from build123d import *

# Parameters (mm, degrees)
F0_R     = 10.0711
F0_R_2   = 9.0551
F1_DEPTH = 1.27
F2_R     = 0.50799


# Not quite as in the source:
# - a fillet or chamfer is up to 0.001 mm smaller than in the source, because OpenCascade refuses the exact size


with BuildPart() as f1:
    # F0 (on Front) → F1 (new body, symmetric)
    with BuildSketch(Plane.XZ):
        Circle(F0_R)
        Circle(F0_R_2, mode=Mode.SUBTRACT)
    extrude(amount=F1_DEPTH, both=True)

    # F2 (radius 0.508 in the source; OpenCascade refuses exactly that, so slightly less here)
    f2_edges = [f1.edges().sort_by_distance(p)[0] for p in [
        (-9.0551, -1.27, 0),
        (-9.0551, 1.27, 0),
        (-10.0711, -1.27, 0),
        (-10.0711, 1.27, 0),
        (10.0711, 0, 0),
    ]]
    fillet(f2_edges, radius=F2_R)


solid = f1.part
The model under review builds one solid part; all positions refer to its coordinate system, in mm. Round coordinates to 2 decimals unless told otherwise and drop trailing zeros. Order: outer loops, then holes, each group sorted by start corner. A loop starts at its lowest first (then second) coordinate and runs counter-clockwise, first axis right, second up. Notation, with made-up numbers: (-32.75, 69.25) - (-15.75, 69.25) arc R38 cw to (-15.75, 108.25) - close; hole circle Ø6 at (-39.75, -37.75). An arc over 180 degrees is marked (long way). Use one line per item in the form item = value.
Q1. Mouldability with a two-part tool opening along Z and no side actions: class faces 1 (the cylindrical face through (-1.96, 0.01, -8.84)), 2 (the cylindrical face through (-1.311, -0.011, 9.985)) as pulls with the +Z half, pulls with the -Z half, needs draft (parallel to the pull), parting line crosses it, or undercut.
Response values:
face_1 = undercut
face_2 = parting line crosses it
Q2. Add section C-C on y = -0.05. Give the boundary of the cut face in (x, z), then the cut area to 3 significant figures.
Response values:
outline = circle Ø20.14 at (0, 0); hole circle Ø18.11 at (0, 0)
area = 61.0 mm^2
Q3. To check wall thickness, follow line 1 (Z direction, x = 0, y = 0.1); line 2 (X direction, y = -0.4, z = -6.25); line 3 (Z direction, x = 7, y = 0.7). State the ranges of each line that lie inside material, in increasing order.
Response values:
line_1 = -10.07 to -9.06, 9.06 to 10.07
line_2 = -7.9 to -6.55, 6.55 to 7.9
line_3 = -7.24 to -5.74, 5.74 to 7.24
Q4. Clearance check with flat-ended pins moving along their axes: P1, Ø1.5, axis at y = 0.5, z = 7.5, coming from the -X side; P2, Ø1.5, axis at x = -7, y = 0.5, coming from the +Z side; P3, Ø3, axis at x = 4, z = -5, coming from the +Y side; P4, Ø1, axis at y = -1, z = 7, coming from the +X side. State where each tip first meets the part, or that it passes through.
Response values:
P1 = -7.47
P2 = 7.9
P3 = through
P4 = 7.66
